Can you work these out from the model? Positions are in its coordinate system, mm. Face numbers are marked on the shaded views. A direction names the side the tool comes from. Round coordinates to 2 decimals unless told otherwise and drop trailing zeros. Order: outer loops, then holes, each group sorted by start corner. A loop starts at its lowest first (then second) coordinate and runs counter-clockwise, first axis right, second up. Notation, with made-up numbers: (-16.75, -11) -> (15.25, -11) arc R5 ccw to (15.25, -3) -> close; hole circle Ø11 at (56.25, 32). An arc over 180 degrees is marked (long way). Use a Markdown table: item, result. Add a question column.
Q1. If we section it at D-D on y = -7.5: List the corners of the cut face in (x, z) for me.
Q2. If we section it at B-B on y = -56: List the corners of the cut face in (x, z) for me.
Q3. If we section it at A-A on z = 50: List the corners of the cut face in (x, y) for me.
Q4. I need wall thicknesses on line 1 along X through (y, z) = (-31, 159); line 2 along Z through (x, y) = (-17, -95.5); line 3 along Y through (x, z) = (-36.5, 188). Which ranges of each line are inside material? Lowest first, please. Write a range as [from, to].
Q5. If we section it at C-C on x = -35.5: List the corners of the cut face in (y, z) for me, plus the area to 3 significant figures.
Q6. For the marked faces 1, 2, 3, 4 and 5, which set-ups out of +Z, -Z, +X, -X, +Y, -Y let a thin tool reach every point of the face, with its end or its side?
Q7. I'm going to push flat-ended pins straight in: pin 1 Ø20.5 at (x, z) = (23.5, 90.5) entering from -Y; pin 2 Ø3 at (y, z) = (-29, 9) entering from +X (3 decimals); pin 3 Ø20.5 at (x, z) = (20, 99) entering from +Y; pin 4 Ø4 at (x, z) = (3.5, 172) entering from +Y. Where does each tip first touch, or does it pass through?
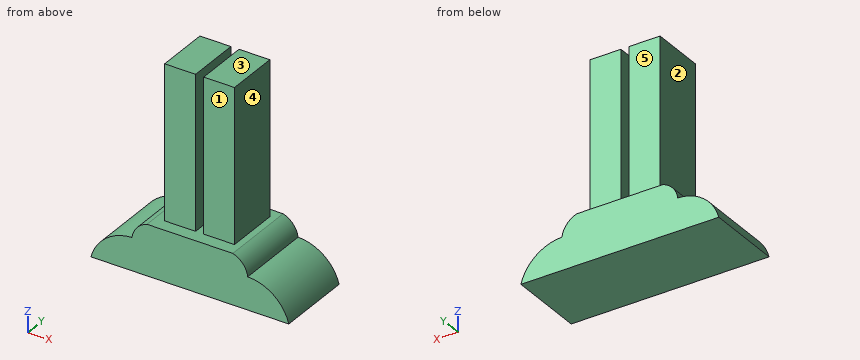
```python
from build123d import *

# Parameters (mm, degrees)
F1_DEPTH = 101.6
F2_W     = 41.042692
F2_H     = 71.251595
F2_W_2   = 40.773873
F3_DEPTH = 203.2


with BuildPart() as f1:
    # F0 (on Front) → F1 (new body)
    with BuildSketch(Plane.XZ):
        with BuildLine():
            Line((-131.095514, -43.026961), (-122.749157, -43.026961))
            Line((-122.749157, -43.026961), (131.095514, -43.026961))
            ThreePointArc((131.095514, -43.026961), (111.101538, -12.406508), (76.700233, 0))
            ThreePointArc((76.700233, 0), (70.237943, 14.771668), (56.841634, 23.743974))
            Line((56.841634, 23.743974), (-56.841634, 23.743974))
            ThreePointArc((-56.841634, 23.743974), (-70.237943, 14.771668), (-76.700233, 0))
            ThreePointArc((-76.700233, 0), (-111.101538, -12.406508), (-131.095514, -43.026961))
        make_face()
    extrude(amount=F1_DEPTH)

    # F2 (on face) → F3 (join)
    with BuildSketch(Plane.XY.offset(23.743974)):
        with Locations((-23.989629, -49.085791)):
            Rectangle(F2_W, F2_H)
        with Locations((27.691657, -49.085791)):
            Rectangle(F2_W_2, F2_H)
    extrude(amount=F3_DEPTH)


solid = f1.part
```
Answer below:
| question | item | result |
|---|---|---|
| 1 | outline | (-131.1, -43.03) -> (131.1, -43.03) arc R57.59 ccw to (76.7, 0) arc R28.76 ccw to (56.84, 23.74) -> (-56.84, 23.74) arc R28.76 ccw to (-76.7, 0) arc R57.59 ccw to start |
| 2 | outline | (-131.1, -43.03) -> (131.1, -43.03) arc R57.59 ccw to (76.7, 0) arc R28.76 ccw to (56.84, 23.74) -> (48.08, 23.74) -> (48.08, 226.94) -> (7.3, 226.94) -> (7.3, 23.74) -> (-3.47, 23.74) -> (-3.47, 226.94) -> (-44.51, 226.94) -> (-44.51, 23.74) -> (-56.84, 23.74) arc R28.76 ccw to (-76.7, 0) arc R57.59 ccw to start |
| 3 | outline | (-44.51, -84.71) -> (-3.47, -84.71) -> (-3.47, -13.46) -> (-44.51, -13.46) -> close; (7.3, -84.71) -> (48.08, -84.71) -> (48.08, -13.46) -> (7.3, -13.46) -> close |
| 4 | line 1 | [-44.51, -3.47], [7.3, 48.08] |
| 4 | line 2 | [-43.03, 23.74] |
| 4 | line 3 | [-84.71, -13.46] |
| 5 | outline | (-101.6, -43.03) -> (0, -43.03) -> (0, 23.74) -> (-13.46, 23.74) -> (-13.46, 226.94) -> (-84.71, 226.94) -> (-84.71, 23.74) -> (-101.6, 23.74) -> close |
| 5 | area | 21,300 mm² |
| 6 | face 1 | +Z, +X, -X, -Y |
| 6 | face 2 | +Z, -X, +Y, -Y |
| 6 | face 3 | +Z, +X, -X, +Y, -Y |
| 6 | face 4 | +Z, +X, +Y, -Y |
| 6 | face 5 | +Z, +X, -X, +Y |
| 7 | pin 1 | y = -84.71 |
| 7 | pin 2 | x = 74.675 |
| 7 | pin 3 | y = -13.46 |
| 7 | pin 4 | through |
